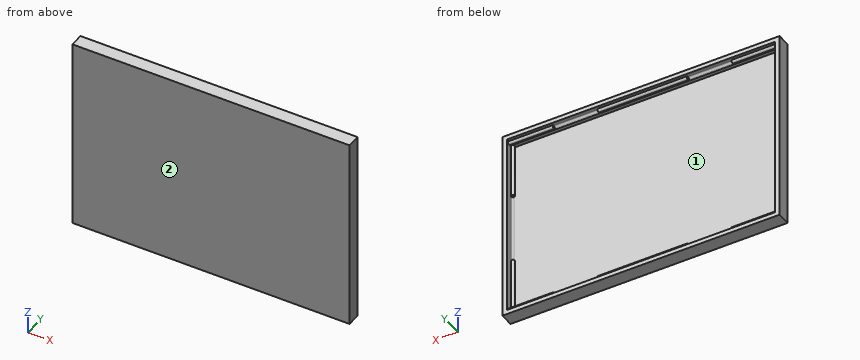
```python
from build123d import *

# Parameters (mm, degrees)
SKETCH_1_W           = 310
SKETCH_1_H           = 220
EXTRUDE_1_DEPTH      = 15
SKETCH_2_W           = 300
SKETCH_2_H           = 210
CUT_EXTRUDE_4_DEPTH  = 6
SKETCH_6_W           = 300
SKETCH_6_H           = 2
EXTRUDE_3_DEPTH      = 2
SKETCH_8_R           = 2
CUT_EXTRUDE_5_DEPTH  = 300
SKETCH_8_2_R         = 2
SKETCH_8_2_R_2       = 1.5
EXTRUDE_1_2_DEPTH    = 300
SKETCH_10_R          = 2
CUT_EXTRUDE_6_DEPTH  = 300
SKETCH_10_2_R        = 2
SKETCH_10_2_R_2      = 1.5
EXTRUDE_2_DEPTH      = 300
SKETCH_12_R          = 2
CUT_EXTRUDE_7_DEPTH  = 50
SKETCH_13_R          = 2
CUT_EXTRUDE_8_DEPTH  = 50
SKETCH_15_W          = 300
SKETCH_15_H          = 202
CUT_EXTRUDE_9_DEPTH  = 4
SKETCH_16_W          = 2
SKETCH_16_H          = 202
EXTRUDE_4_DEPTH      = 2
SKETCH_14_R          = 2
CUT_EXTRUDE_10_DEPTH = 202
SKETCH_14_2_R        = 2
SKETCH_14_2_R_2      = 1.5
EXTRUDE_3_2_DEPTH    = 202
SKETCH_18_R          = 2
CUT_EXTRUDE_11_DEPTH = 80


with BuildPart() as part:
    # 草图1 → Extrude 1 (new body)
    with BuildSketch(Plane(origin=(0, 0, 0), x_dir=(1, 0, 0), z_dir=(0, 1, 0))):
        with Locations((0.660377358, 22.830188679)):
            Rectangle(SKETCH_1_W, SKETCH_1_H)
    extrude(amount=EXTRUDE_1_DEPTH)

    # 草图2 → 切除-拉伸4 (cut)
    with BuildSketch(Plane(origin=(0, 15, 0), x_dir=(1, 0, 0), z_dir=(0, 1, 0))):
        with Locations((0.660377358, 22.830188679)):
            Rectangle(SKETCH_2_W, SKETCH_2_H)
    extrude(amount=-CUT_EXTRUDE_4_DEPTH, mode=Mode.SUBTRACT)

    # 草图6 → Extrude 3 (add)
    with BuildSketch(Plane(origin=(0, 9, 0), x_dir=(1, 0, 0), z_dir=(0, 1, 0))):
        with Locations((0.660377358, 126.830188679)):
            Rectangle(SKETCH_6_W, SKETCH_6_H)
        with Locations((0.660377358, -81.169811321)):
            Rectangle(SKETCH_6_W, SKETCH_6_H)
    extrude(amount=EXTRUDE_3_DEPTH)

    # 草图8 → 切除-拉伸5 (cut)
    with BuildSketch(Plane(origin=(150.660377358, 0, 0), x_dir=(0, 0, -1), z_dir=(1, 0, 0))):
        with Locations((-80.169811321, 11)):
            Circle(SKETCH_8_R)
    extrude(amount=-CUT_EXTRUDE_5_DEPTH, mode=Mode.SUBTRACT)

    # 草图8<2> → Extrude 1 2 (add)
    with BuildSketch(Plane(origin=(150.660377358, 0, 0), x_dir=(0, 0, -1), z_dir=(1, 0, 0))):
        with Locations((-80.169811321, 11)):
            Circle(SKETCH_8_2_R)
        with Locations((-80.169811321, 11)):
            Circle(SKETCH_8_2_R_2, mode=Mode.SUBTRACT)
    extrude(amount=-EXTRUDE_1_2_DEPTH)

    # 草图10 → 切除-拉伸6 (cut)
    with BuildSketch(Plane(origin=(150.660377358, 0, 0), x_dir=(0, 0, -1), z_dir=(1, 0, 0))):
        with Locations((125.830188679, 11)):
            Circle(SKETCH_10_R)
    extrude(amount=-CUT_EXTRUDE_6_DEPTH, mode=Mode.SUBTRACT)

    # 草图10<2> → 拉伸-薄壁2 (add)
    with BuildSketch(Plane(origin=(150.660377358, 0, 0), x_dir=(0, 0, -1), z_dir=(1, 0, 0))):
        with Locations((125.830188679, 11)):
            Circle(SKETCH_10_2_R)
        with Locations((125.830188679, 11)):
            Circle(SKETCH_10_2_R_2, mode=Mode.SUBTRACT)
    extrude(amount=-EXTRUDE_2_DEPTH)

    # 草图12 → 切除-拉伸7 (cut)
    with BuildSketch(Plane(origin=(100.660377358, 0, 0), x_dir=(0, 0, -1), z_dir=(1, 0, 0))):
        with Locations((-80.169811321, 11)):
            Circle(SKETCH_12_R)
        with Locations((125.830188679, 11)):
            Circle(SKETCH_12_R)
    extrude(amount=-CUT_EXTRUDE_7_DEPTH, mode=Mode.SUBTRACT)

    # 草图13 → 切除-拉伸8 (cut)
    with BuildSketch(Plane(origin=(-49.339622642, 0, 0), x_dir=(0, 0, -1), z_dir=(1, 0, 0))):
        with Locations((-80.169811321, 11)):
            Circle(SKETCH_13_R)
        with Locations((125.830188679, 11)):
            Circle(SKETCH_13_R)
    extrude(amount=-CUT_EXTRUDE_8_DEPTH, mode=Mode.SUBTRACT)

    # 草图15 → 切除-拉伸9 (cut)
    with BuildSketch(Plane(origin=(0, 9, 0), x_dir=(1, 0, 0), z_dir=(0, 1, 0))):
        with Locations((0.660377358, 22.830188679)):
            Rectangle(SKETCH_15_W, SKETCH_15_H)
    extrude(amount=-CUT_EXTRUDE_9_DEPTH, mode=Mode.SUBTRACT)

    # 草图16 → 凸台-拉伸4 (add)
    with BuildSketch(Plane(origin=(0, 5, 0), x_dir=(1, 0, 0), z_dir=(0, 1, 0))):
        with Locations((-148.339622642, 22.830188679)):
            Rectangle(SKETCH_16_W, SKETCH_16_H)
        with Locations((149.660377358, 22.830188679)):
            Rectangle(SKETCH_16_W, SKETCH_16_H)
    extrude(amount=EXTRUDE_4_DEPTH)

    # 草图14 → 切除-拉伸10 (cut)
    with BuildSketch(Plane.XY.offset(78.169811321)):
        with Locations((-147.339622642, 7)):
            Circle(SKETCH_14_R)
        with Locations((148.660377358, 7)):
            Circle(SKETCH_14_R)
    extrude(amount=-CUT_EXTRUDE_10_DEPTH, mode=Mode.SUBTRACT)

    # 草图14<2> → Extrude 3 2 (add)
    # profile 1 of 2: a face of its own
    with BuildSketch(Plane.XY.offset(78.169811321)):
        with Locations((-147.339622642, 7)):
            Circle(SKETCH_14_2_R)
        with Locations((-147.339622642, 7)):
            Circle(SKETCH_14_2_R_2, mode=Mode.SUBTRACT)
    # profile 2 of 2: a face of its own
    with BuildSketch(Plane.XY.offset(78.169811321)):
        with Locations((148.660377358, 7)):
            Circle(SKETCH_14_2_R)
        with Locations((148.660377358, 7)):
            Circle(SKETCH_14_2_R_2, mode=Mode.SUBTRACT)
    extrude(amount=-EXTRUDE_3_2_DEPTH)

    # 草图18 → 切除-拉伸11 (cut)
    with BuildSketch(Plane.XY.offset(17.169811321)):
        with Locations((-147.339622642, 7)):
            Circle(SKETCH_18_R)
        with Locations((148.660377358, 7)):
            Circle(SKETCH_18_R)
    extrude(amount=-CUT_EXTRUDE_11_DEPTH, mode=Mode.SUBTRACT)


solid = part.part
```
Build history of the part. All positions in model axes, mm. Face numbers are marked on the shaded views. Give positions to 0.01 mm unless a question says otherwise; leave off trailing zeros. Loops run counter-clockwise (first coordinate to the right, second up) from the corner with the lowest first, then second, coordinate; pieces in that order, holes last.
1) Band-saw the part on A-A on x = -33. List the corners of the cut face in (y, z).
Values follow:
outline: (0, -132.83) - (15, -132.83) - (15, -127.83) - (11, -127.83) arc R2 ccw (long way) to (9, -125.83) - (9, -123.83) - (5, -123.83) - (5, 78.17) - (9, 78.17) - (9, 80.17) arc R2 ccw (long way) to (11, 82.17) - (15, 82.17) - (15, 87.17) - (0, 87.17) - close; hole circle Ø3 at (11, -125.83); hole circle Ø3 at (11, 80.17)
2) Two-plate mould, pull along Z, no slides. Class the marked faces 1 and 2: released by +Z, released by -Z, zero draft, split by the parting line, or undercut.
Values follow:
face 1: undercut
face 2: zero draft
3) Drop flat-ended pins along their axis: P1, Ø12, axis at x = 28, z = 28.5, coming from the +Y side; P2, Ø1, axis at x = 38, z = -124.5, coming from the +Y side. Give the stop position or say it passes through.
Values follow:
P1: stops at y = 5
P2: stops at y = 12.82
4) Band-saw the part on B-B on z = 42. List the corners of the cut face in (x, y), then the cut area to 3 significant figures.
Values follow:
outline: (-154.34, 0) - (155.66, 0) - (155.66, 15) - (150.66, 15) - (150.66, 7) arc R2 ccw (long way) to (148.66, 5) - (-147.34, 5) arc R2 ccw (long way) to (-149.34, 7) - (-149.34, 15) - (-154.34, 15) - close; hole circle Ø3 at (-147.34, 7); hole circle Ø3 at (148.66, 7)
area: 1,660 mm2
5) Band-saw the part on D-D on x = 60.5. List the corners of the cut face in (y, z).
Values follow:
outline: (0, -132.83) - (15, -132.83) - (15, -127.83) - (11, -127.83) arc R2 cw to (9, -125.83) - (9, -123.83) - (5, -123.83) - (5, 78.17) - (9, 78.17) - (9, 80.17) arc R2 cw to (11, 82.17) - (15, 82.17) - (15, 87.17) - (0, 87.17) - close
6) Band-saw the part on C-C on z = -54. List the corners of the cut face in (x, y).
Values follow:
outline: (-154.34, 0) - (155.66, 0) - (155.66, 15) - (150.66, 15) - (150.66, 7) arc R2 cw to (148.66, 5) - (-147.34, 5) arc R2 cw to (-149.34, 7) - (-149.34, 15) - (-154.34, 15) - close
7) Probe line 1 along X through (y, z) = (12.5, -105); line 2 along Z through (x, y) = (62, 5.25); line 3 along Z through (x, y) = (1, 13.5). List the from-to ranges inside material, lowest first.
Values follow:
line 1: x = -154.34 to -149.34, 150.66 to 155.66
line 2: z = -132.83 to -123.83, 78.17 to 87.17
line 3: z = -132.83 to -127.83, 82.17 to 87.17
